Autodesk Inventor part; units mm, degrees
ref_plane "YZ Plane" through (0, 0, 0) normal (1, 0, 0) x (0, 1, 0)
ref_plane "XZ Plane" through (0, 0, 0) normal (0, 1, 0) x (-1, 0, 0)
ref_plane "XY Plane" through (0, 0, 0) normal (0, 0, 1) x (1, 0, 0)
sketch "Sketch1" plane through (0, 0, 0) normal (0, 0, 1) x (1, 0, 0)
  line L0 (-136.0714, 83.0036) -> (16.3286, -18.5964)
  line L1 (16.3286, -18.5964) -> (67.1286, -18.5964)
  line L2 (67.1286, -18.5964) -> (67.1286, 184.6036)
  line L3 (67.1286, 184.6036) -> (-136.0714, 184.6036)
  line L4 (-136.0714, 184.6036) -> (-136.0714, 83.0036)
  point P0 (0, 0)
  dimension "d0" = 101.6
  dimension "d1" = 50.8
  dimension "d2" = 203.2
  dimension "d4" = 203.2
extrude "Extrusion1" add sketch "Sketch1" along normal blind 4.7625
sketch "Sketch2" plane through (0, 0, 4.7625) normal (0, 0, 1) x (1, 0, 0)
  line L0 (16.3286, -18.5964) -> (67.1286, -18.5964)
  line L1 (67.1286, -18.5964) -> (67.1286, 184.6036)
  line L2 (67.1286, 184.6036) -> (-136.0714, 184.6036)
  line L3 (-136.0714, 184.6036) -> (-136.0714, 83.0036)
  point P0 (0, 0)
  point P1 (-123.3714, 171.9036)
  point P2 (-97.9714, 171.9036)
  point P3 (-72.5714, 171.9036)
  point P4 (-47.1714, 171.9036)
  point P5 (-21.7714, 171.9036)
  point P6 (3.6286, 171.9036)
  point P7 (29.0286, 171.9036)
  point P8 (54.4286, 171.9036)
  point P9 (-123.3714, 146.5036)
  point P10 (-97.9714, 146.5036)
  point P11 (-72.5714, 146.5036)
  point P12 (-47.1714, 146.5036)
  point P13 (-21.7714, 146.5036)
  point P14 (3.6286, 146.5036)
  point P15 (29.0286, 146.5036)
  point P16 (54.4286, 146.5036)
  point P17 (-123.3714, 121.1036)
  point P18 (-97.9714, 121.1036)
  point P19 (-72.5714, 121.1036)
  point P20 (-47.1714, 121.1036)
  point P21 (-21.7714, 121.1036)
  point P22 (3.6286, 121.1036)
  point P23 (29.0286, 121.1036)
  point P24 (54.4286, 121.1036)
  point P25 (-123.3714, 95.7036)
  point P26 (-97.9714, 95.7036)
  point P27 (-72.5714, 95.7036)
  point P28 (-47.1714, 95.7036)
  point P29 (-21.7714, 95.7036)
  point P30 (3.6286, 95.7036)
  point P31 (29.0286, 95.7036)
  point P32 (54.4286, 95.7036)
  point P33 (54.4286, 70.3036)
  point P34 (54.4286, 44.9036)
  point P35 (54.4286, 19.5036)
  point P36 (54.4286, -5.8964)
  point P37 (29.0286, 95.7036)
  point P38 (29.0286, 70.3036)
  point P39 (29.0286, 44.9036)
  point P40 (29.0286, 19.5036)
  point P41 (29.0286, -5.8964)
  dimension "d26" = 12.7
  dimension "d27" = 12.7
  dimension "d30" = 25.4
  dimension "d33" = 25.4
  dimension "d38" = 25.4
  dimension "d41" = 25.4
hole "Hole1" at (-123.3714, 171.9036, 4.7625) at (-97.9714, 171.9036, 4.7625) at (-72.5714, 171.9036, 4.7625) at (-47.1714, 171.9036, 4.7625) at (-21.7714, 171.9036, 4.7625) at (3.6286, 171.9036, 4.7625) at (29.0286, 171.9036, 4.7625) at (54.4286, 171.9036, 4.7625) at (-123.3714, 146.5036, 4.7625) at (-97.9714, 146.5036, 4.7625) at (-72.5714, 146.5036, 4.7625) at (-47.1714, 146.5036, 4.7625) at (-21.7714, 146.5036, 4.7625) at (3.6286, 146.5036, 4.7625) at (29.0286, 146.5036, 4.7625) at (54.4286, 146.5036, 4.7625) at (-123.3714, 121.1036, 4.7625) at (-97.9714, 121.1036, 4.7625) at (-72.5714, 121.1036, 4.7625) at (-47.1714, 121.1036, 4.7625) at (-21.7714, 121.1036, 4.7625) at (3.6286, 121.1036, 4.7625) at (29.0286, 121.1036, 4.7625) at (54.4286, 121.1036, 4.7625) at (-123.3714, 95.7036, 4.7625) at (-97.9714, 95.7036, 4.7625) at (-72.5714, 95.7036, 4.7625) at (-47.1714, 95.7036, 4.7625) at (-21.7714, 95.7036, 4.7625) at (3.6286, 95.7036, 4.7625) at (29.0286, 95.7036, 4.7625) at (54.4286, 95.7036, 4.7625) at (54.4286, 70.3036, 4.7625) at (54.4286, 44.9036, 4.7625) at (54.4286, 19.5036, 4.7625) at (54.4286, -5.8964, 4.7625) at (29.0286, 70.3036, 4.7625) at (29.0286, 44.9036, 4.7625) at (29.0286, 19.5036, 4.7625) at (29.0286, -5.8964, 4.7625) direction (0, 0, -1) diameter 6.35 end through all
sketch "Sketch3" plane through (0, 0, 0) normal (0, 0, -1) x (-1, 0, 0)
  line L0 (136.0714, 83.0036) -> (-16.3286, -18.5964)
  line L1 (33.684, 65.5453) -> (109.884, 65.5453)
  line L2 (33.684, 65.5453) -> (33.684, 14.7453)
  point P0 (0, 0)
  dimension "d53" = 50.8
  dimension "d54" = 33.3417
  dimension "d55" = 76.2
extrude "Extrusion2" cut sketch "Sketch3" against normal blind 25.4
equation "\"d4\" = d2"
properties part number "2020-2040_mounting_plate"
Read the model definition and answer for the solid it produces. Units are mm, in the model's axes. A direction names the side the tool comes from. Round coordinates to 2 decimals unless told otherwise and drop trailing zeros. Write each loop counter-clockwise with the first axis right and the second up, starting at its lowest first coordinate (ties: lowest second). Pieces come first, ordered by that corner, then holes.
1. Determine the mould class of faces 3 (the face through (-36, 107, 4.762)), 4 (the face through (-9.03, -1.69, 2.35)), 5 (the face through (28.889, 149.676, 2.348)), 6 (the face through (52.28, 148.84, 2.35)) for opening direction Y: pulls with the +Y half, pulls with the -Y half, needs draft (parallel to the pull), parting line crosses it, or undercut.
2. The part is cut by section B-B, the plane x = -37. Determine the outline of the cut face in (y, z).
3. The part is cut by section C-C, the plane z = 2.05. State how many separate pieces and enclosed holes the cut face has, then the cut area to 3 significant figures.
4. The part is cut by section A-A, the plane y = 54.5. Determine the outline of the cut face in (x, z), then the cut area to 3 significant figures.
5. Straight lines are drawn through the part: L1, parallel to X at y = 47, z = 3.45; L2, parallel to X at y = -3, z = 0.5; L3, parallel to Y at x = -88, z = 1.7. For each, find the intervals that lie inside material, in ascending order.
6. Which of the six approach directions +Z, -Z, +X, -X, +Y, -Y give full straight-line access (tool end or side, diameter ignored) to faces 1 (the face through (28.889, 22.676, 2.348)), 2 (the face through (-71, 65.545, 2))?
7. Given pin 1 Ø8.5 at (x, y) = (29.03, 121.1) entering from -Z; pin 2 Ø1.5 at (x, z) = (-70.5, 2) entering from -Y, each flat-ended and moving along its own axis, determine where each tip first touches the part or whether it passes through.
Values:
1. face 3: needs draft
1. face 4: pulls with the -Y half
1. face 5: undercut
1. face 6: undercut
2. outline: (65.55, 0) - (184.6, 0) - (184.6, 4.76) - (65.55, 4.76) - close
3. separate pieces: 1
3. enclosed holes: 40
3. area: 30,300 mm2
4. outline: (-33.68, 0) - (67.13, 0) - (67.13, 4.76) - (-33.68, 4.76) - close
4. area: 480 mm2
5. L1: x = -33.68 to 26.64, 31.41 to 52.04, 56.81 to 67.13
5. L2: x = -7.07 to 27.73, 30.33 to 53.13, 55.73 to 67.13
5. L3: y = 65.55 to 184.6
6. face 1: +Z, -Z
6. face 2: +Z, -Z, -X, -Y
7. pin 1: stops at z = 0
7. pin 2: stops at y = 65.55
